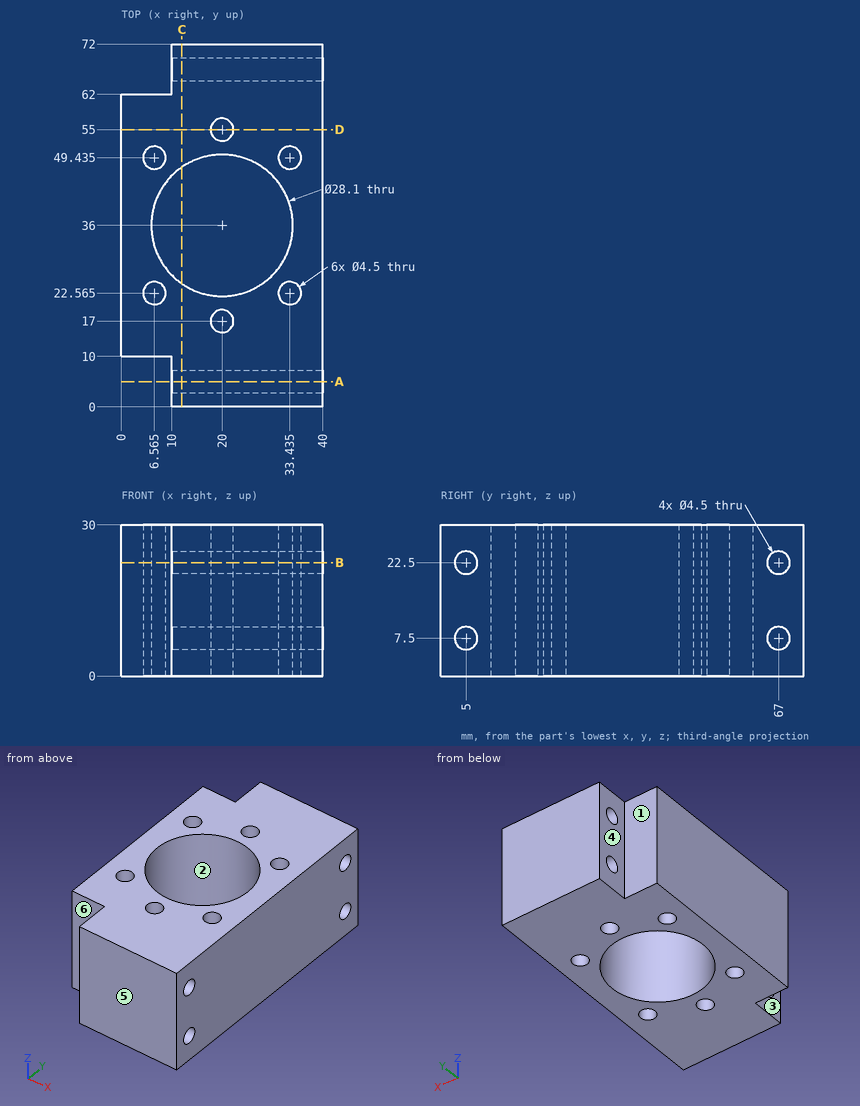
Check sheet for the drawn part. Datum: minimum x, y, z corner. Units: mm. A direction names the side the tool comes from. Give positions to 0.01 mm unless a question says otherwise; leave off trailing zeros. Loops run counter-clockwise (first coordinate to the right, second up) from the corner with the lowest first, then second, coordinate; pieces in that order, holes last. Notation, with made-up numbers: M -20,47 L 17,47 A13 cw 17,70 Z; hole C 10,63 d11. An arc over 180 degrees is marked long. Return JSON: item names as keys, results as strings.
1) Section check C-C, the plane x = 12. Enter the section's corners in (y, z).
Findings:
{"outline": "M 0,0 L 24.45,0 L 24.45,30 L 0,30 Z; M 47.55,0 L 72,0 L 72,30 L 47.55,30 Z; hole C 5,7.5 d4.5; hole C 5,22.5 d4.5; hole C 67,7.5 d4.5; hole C 67,22.5 d4.5"}
2) Mould release check, pull along Y, two halves, no side actions. Record for the marked faces 1, 2 and 3: released by +Y, released by -Y, zero draft, split by the parting line, or undercut.
Findings:
{"face 1": "released by +Y", "face 2": "undercut", "face 3": "zero draft"}
3) Section check B-B, the plane z = 22.5. Count the separate pieces of the cut face and the enclosed holes in it, and give its area (3 significant figures).
Findings:
{"separate pieces": "3", "enclosed holes": "7", "area": "1,690 mm2"}
4) Section check A-A, the plane y = 5. Enter the section's corners in (x, z).
Findings:
{"outline": "M 10,0 L 40,0 L 40,5.25 L 10,5.25 Z; M 10,9.75 L 40,9.75 L 40,20.25 L 10,20.25 Z; M 10,24.75 L 40,24.75 L 40,30 L 10,30 Z"}
5) Material ranges on L1, parallel to Y at x = 20, z = 7.5; L2, parallel to Z at x = 30.5, y = 67; L3, parallel to Y at x = 20, z = 13, recorded low to high. Write a range as [from, to].
Findings:
{"L1": "y = [0, 2.75], [7.25, 14.75], [19.25, 21.95], [50.05, 52.75], [57.25, 64.75], [69.25, 72]", "L2": "z = [0, 5.25], [9.75, 20.25], [24.75, 30]", "L3": "y = [0, 14.75], [19.25, 21.95], [50.05, 52.75], [57.25, 72]"}
6) Gauge pin test, flat ends, axial feed: P1, Ø6, axis at y = 67, z = 7.5, coming from the -X side; P2, Ø11, axis at x = 3, z = 13, coming from the +Y side. Record the tip position at first contact, or that the pin passes through.
Findings:
{"P1": "stops at x = 10", "P2": "stops at y = 62"}
7) Section check D-D, the plane y = 55. Enter the section's corners in (x, z), and give its area (4 significant figures).
Findings:
{"outline": "M 0,0 L 17.75,0 L 17.75,30 L 0,30 Z; M 22.25,0 L 40,0 L 40,30 L 22.25,30 Z", "area": "1,065 mm2"}
8) Tool access check on the marked faces 4, 5 and 6. Record the directions out of +Z, -Z, +X, -X, +Y, -Y that give a thin tool (end or side, any length) a straight path to the whole face; none if there is none.
Findings:
{"face 4": "+Z, -Z, -X, +Y", "face 5": "+Z, -Z, +X, -X, -Y", "face 6": "+Z, -Z, -X, -Y"}
